Check sheet for the drawn part. Datum: minimum x, y, z corner. Units: mm. Coordinates: 2 decimals unless noted, no trailing zeros. Order: outer loops, then holes, each group sorted by start corner. A loop starts at its lowest first (then second) coordinate and runs counter-clockwise, first axis right, second up. Notation, with made-up numbers: M 29,-2 L 63,-2 A15 ccw 63,19 Z; hole C 29.25,35.5 d3. An arc over 180 degrees is marked long. Return JSON: item names as keys, results as strings. Group by question number.
Q1. Thickness scan on probe 1 along X at (y, z) = (2.25, 82.55); probe 2 along X at (y, z) = (2.05, 5.08); probe 3 along Z at (x, y) = (9.5, 0.65). Record the ranges inside material, lowest first.
Q2. Go/stop test with flat-tipped pins: pin 1 Ø3 at (x, z) = (51.816, 5.08) entering from -Y; pin 2 Ø5.5 at (x, z) = (72.771, 82.55) entering from +Y. Record where each tip stops, or that it passes through.
Q3. Section check B-B, the plane y = 3.25. Count the separate pieces of the cut face and the enclosed holes in it, then the cut area to 3 significant figures.
Q4. Section check A-A, the plane z = 82.55. Enter the section's corners in (x, y).
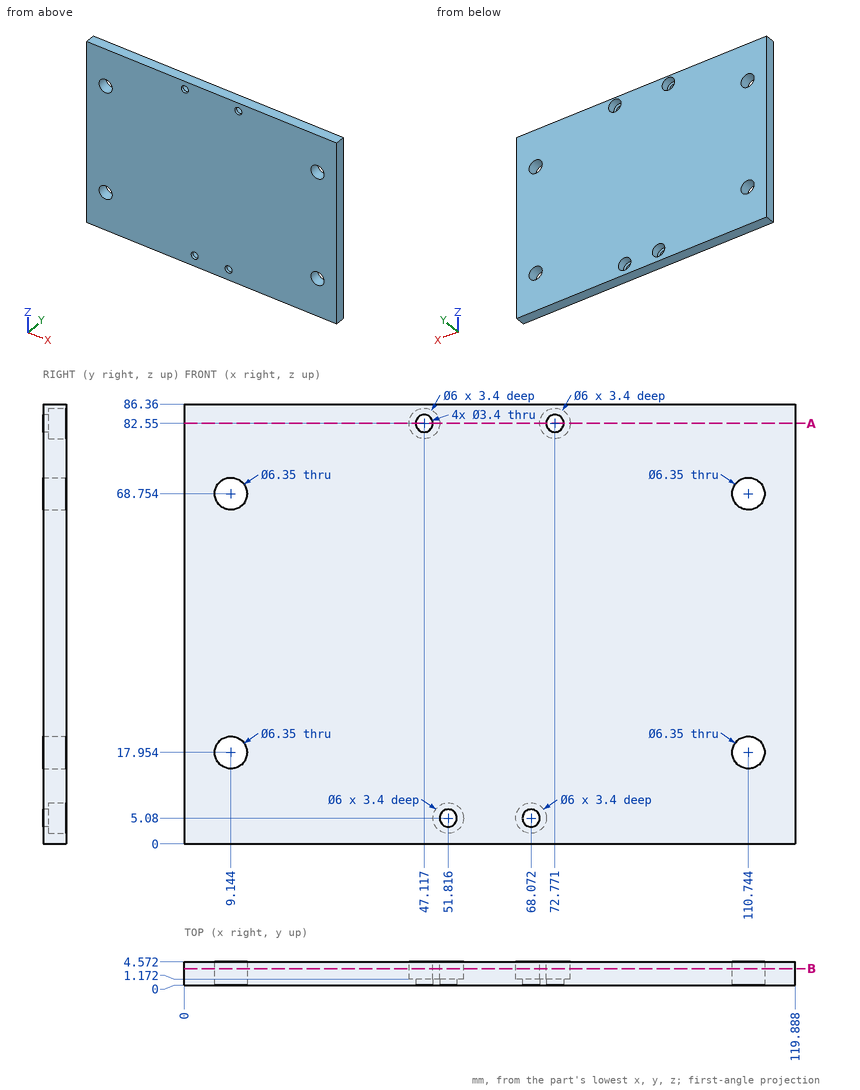
Numbers:
{
 "1": {"probe 1": "x = 0 to 44.12, 50.12 to 69.77, 75.77 to 119.89", "probe 2": "x = 0 to 48.82, 54.82 to 65.07, 71.07 to 119.89", "probe 3": "z = 0 to 14.8, 21.11 to 65.6, 71.91 to 86.36"},
 "2": {"pin 1": "passes through", "pin 2": "stops at y = 1.17"},
 "3": {"separate pieces": "1", "enclosed holes": "8", "area": "10,100 mm2"},
 "4": {"outline": "M 0,0 L 45.42,0 L 45.42,1.17 L 44.12,1.17 L 44.12,4.57 L 0,4.57 Z; M 48.82,0 L 71.07,0 L 71.07,1.17 L 69.77,1.17 L 69.77,4.57 L 50.12,4.57 L 50.12,1.17 L 48.82,1.17 Z; M 74.47,0 L 119.89,0 L 119.89,4.57 L 75.77,4.57 L 75.77,1.17 L 74.47,1.17 Z"}
}
